from build123d import *

# Parameters (mm, degrees)
SKETCH002_R  = 2.5
PAD002_DEPTH = 13
SKETCH_W     = 35
SKETCH_H     = 13
PAD_DEPTH    = 5
SKETCH003_R  = 3.3
PAD003_DEPTH = 13
SKETCH004_R  = 5
POCKET_DEPTH = 5


with BuildPart() as pad002:
    # Sketch002 → Pad002 (new body)
    with BuildSketch(Plane.XZ.offset(6.5)):
        with Locations((17.683945, 2.483897)):
            Circle(SKETCH002_R)
    extrude(amount=-PAD002_DEPTH)


with BuildPart() as part_mirroring001:
    # Part__Mirroring001: instance of Pad002
    add(pad002.part.mirror(Plane(origin=(0, 0, 2.483897), x_dir=(0, -1, 0), z_dir=(1, 0, 0))))


with BuildPart() as scassi:
    # Fusion001 base: copy of Pad002
    add(pad002.part)

    # Fusion001: union Part__Mirroring001
    add(part_mirroring001.part)


with BuildPart() as pocket:
    # Sketch → Pad (new body)
    with BuildSketch(Plane.XY):
        Rectangle(SKETCH_W, SKETCH_H)
    extrude(amount=PAD_DEPTH)

    # Sketch003 → Pad003 (new body)
    with BuildSketch(Plane.XZ.offset(6.5)):
        with Locations((17.683945, 2.483897)):
            Circle(SKETCH003_R)
        with Locations((-17.683945, 2.483897)):
            Circle(SKETCH003_R)
    extrude(amount=-PAD003_DEPTH)

    # Cut: cut scassi
    add(scassi.part, mode=Mode.SUBTRACT)

    # Sketch004 → Pocket (cut)
    with BuildSketch(Plane.XY.offset(5)):
        Circle(SKETCH004_R)
    extrude(amount=-POCKET_DEPTH, mode=Mode.SUBTRACT)


solid = pocket.part
Part model, mm, in its own coordinate system. A direction names the side the tool comes from. Coordinates: 2 decimals unless noted, no trailing zeros. Write each loop counter-clockwise with the first axis right and the second up, starting at its lowest first coordinate (ties: lowest second). Pieces come first, ordered by that corner, then holes. Notation, with made-up numbers: M -14,-15.75 L 35,-15.75 A9 cw 35,-2.75 Z; hole C 3,10 d4. An arc over 180 degrees is marked long. Return JSON: item names as keys, results as strings.
1. Saw through at A-A, the plane x = 0. Write the cut outline in (y, z), then the cut area to 3 significant figures.
Determined:
{"outline": "M -6.5,0 L -5,0 L -5,5 L -6.5,5 Z; M 5,0 L 6.5,0 L 6.5,5 L 5,5 Z", "area": "15.0 mm²"}
2. Pull direction Z, two halves, no side cores. Call faces 3 (the face through (0, -6.5, 3)), 4 (the face through (-15.186, -0.091, 2.594)), 5 (the face through (-4, 4, 0)): pulls with the +Z half, pulls with the -Z half, needs draft (parallel to the pull), parting line crosses it, or undercut.
Determined:
{"face 3": "needs draft", "face 4": "undercut", "face 5": "pulls with the -Z half"}
3. Probe L1, parallel to X at y = 6.25, z = 2.5; L2, parallel to X at y = -2.25, z = 1; L3, parallel to X at y = -2.75, z = 1.5. List the from-to ranges inside material, lowest first.
Determined:
{"L1": "-20.98 to -20.18, -15.18 to 15.18, 20.18 to 20.98", "L2": "-20.63 to -19.7, -15.67 to -4.47, 4.47 to 15.67, 19.7 to 20.63", "L3": "-20.83 to -19.98, -15.39 to -4.18, 4.18 to 15.39, 19.98 to 20.83"}
4. Saw through at B-B, the plane y = 2.5. Write the cut outline in (x, z), then the cut area to 3 significant figures.
Determined:
{"outline": "M -15.55,5 A3.3 ccw long -15.51,0 L -4.33,0 L -4.33,5 Z; M 4.33,0 L 15.51,0 A3.3 ccw long 15.55,5 L 4.33,5 Z; hole C -17.68,2.48 d5; hole C 17.68,2.48 d5", "area": "133 mm²"}
5. Saw through at C-C, the plane z = 1.75. Write the cut outline in (x, y).
Determined:
{"outline": "M -20.9,-6.5 L -20.07,-6.5 L -20.07,6.5 L -20.9,6.5 Z; M -15.29,-6.5 L 15.29,-6.5 L 15.29,6.5 L -15.29,6.5 Z; M 20.07,-6.5 L 20.9,-6.5 L 20.9,6.5 L 20.07,6.5 Z; hole C 0,0 d10"}
6. Flat gauge pins, fed straight in: pin 1 Ø2 at (x, y) = (-11, 2.5) entering from -Z; pin 2 Ø2 at (x, y) = (16, 3) entering from -Z; pin 3 Ø1.5 at (y, z) = (0, 4.5) entering from -X. Where does each tip first touch, or does it go through?
Determined:
{"pin 1": "z = 0", "pin 2": "z = -0.74", "pin 3": "x = -20.73"}
7. Saw through at D-D, the plane y = -0.5. Write the cut outline in (x, z), then the cut area to 3 significant figures.
Determined:
{"outline": "M -15.55,5 A3.3 ccw long -15.51,0 L -4.97,0 L -4.97,5 Z; M 4.97,0 L 15.51,0 A3.3 ccw long 15.55,5 L 4.97,5 Z; hole C -17.68,2.48 d5; hole C 17.68,2.48 d5", "area": "127 mm²"}
8. 3-axis set-ups, long thin cutter, end or side, ignore diameter. For faces 1 (the face through (0, 6.5, 3)), 2 (the face through (-4, 4, 5)): which of +Z, -Z, +X, -X, +Y, -Y reach the whole face in a straight line?
Determined:
{"face 1": "+Z, -Z, +X, -X, +Y", "face 2": "+Z, +Y, -Y"}
